Design review of the part built by this model. Coordinates are the model's own, in mm. A direction names the side the tool comes from. Coordinates: 2 decimals unless noted, no trailing zeros. Order: outer loops, then holes, each group sorted by start corner. A loop starts at its lowest first (then second) coordinate and runs counter-clockwise, first axis right, second up. Notation, with made-up numbers: (-14.75, -19) - (38.25, -19) arc R24 cw to (38.25, 11) - close; hole circle Ø9 at (68, 15.5). An arc over 180 degrees is marked (long way). Write each question's results on one line, items separated by ' | '. Start each with the question number.
```python
from build123d import *

# Parameters (mm, degrees)
F1_DEPTH = 15
F2_R     = 3.5
F3_DEPTH = 4.1
F4_R     = 2.25
F5_DEPTH = 25
F6_W     = 9.15
F6_H     = 11
F7_DEPTH = 52.92131


with BuildPart() as f1:
    # F0 (on Front) → F1 (new body)
    with BuildSketch(Plane.XZ):
        with BuildLine():
            Line((32, 0), (0, 0))
            Line((0, 0), (0, -11))
            ThreePointArc((0, -11), (0.87868, -13.12132), (3, -14))
            Line((3, -14), (6.5, -14))
            ThreePointArc((6.5, -14), (8.62132, -14.87868), (9.5, -17))
            Line((9.5, -17), (9.5, -17.757359))
            ThreePointArc((9.5, -17.757359), (9.728361, -18.90541), (10.37868, -19.87868))
            Line((10.37868, -19.87868), (26.29899, -35.79899))
            ThreePointArc((26.29899, -35.79899), (26.949308, -36.77226), (27.17767, -37.92031))
            Line((27.17767, -37.92031), (27.17767, -41.92031))
            ThreePointArc((27.17767, -41.92031), (28.056349, -44.041631), (30.17767, -44.92031))
            Line((30.17767, -44.92031), (49.92031, -44.92031))
            ThreePointArc((49.92031, -44.92031), (52.041631, -44.041631), (52.92031, -41.92031))
            Line((52.92031, -41.92031), (52.92031, -40.42031))
            ThreePointArc((52.92031, -40.42031), (52.041631, -38.29899), (49.92031, -37.42031))
            Line((49.92031, -37.42031), (44.162951, -37.42031))
            ThreePointArc((44.162951, -37.42031), (43.014901, -37.191949), (42.041631, -36.541631))
            Line((42.041631, -36.541631), (25.37868, -19.87868))
            ThreePointArc((25.37868, -19.87868), (24.728361, -18.90541), (24.5, -17.757359))
            Line((24.5, -17.757359), (24.5, -17))
            ThreePointArc((24.5, -17), (25.37868, -14.87868), (27.5, -14))
            Line((27.5, -14), (29, -14))
            ThreePointArc((29, -14), (31.12132, -13.12132), (32, -11))
            Line((32, -11), (32, 0))
        make_face()
    extrude(amount=F1_DEPTH)

    # F2 (on face) → F3 (cut)
    with BuildSketch(Plane.XZ.offset(15)):
        with Locations((26.5, -6.5)):
            Circle(F2_R)
        with Locations((5.5, -6.5)):
            Circle(F2_R)
    extrude(amount=-F3_DEPTH, mode=Mode.SUBTRACT)

    # F4 (on face) → F5 (cut)
    with BuildSketch(Plane.XZ.offset(15)):
        with Locations((5.5, -6.5)):
            Circle(F4_R)
        with Locations((26.5, -6.5)):
            Circle(F4_R)
    extrude(amount=-F5_DEPTH, mode=Mode.SUBTRACT)

    # F6 (on face) → F7 (cut, through all)
    with BuildSketch(Plane(origin=(0, 0, 0), x_dir=(0, -1, 0), z_dir=(-1, 0, 0))):
        with Locations((4.575, -5.5)):
            Rectangle(F6_W, F6_H)
        with BuildLine():
            ThreePointArc((6, -45), (6.87868, -47.12132), (9, -48))
            Line((9, -48), (15, -48))
            Line((15, -48), (15, -16))
            Line((15, -16), (9, -16))
            ThreePointArc((9, -16), (6.87868, -16.87868), (6, -19))
            Line((6, -19), (6, -45))
        make_face()
    extrude(amount=-F7_DEPTH, mode=Mode.SUBTRACT)


solid = f1.part
```
(1) Take a section at B-B (z = -6.5). State the section outline as (x, y) points.
(2) Clearance check with flat-ended pins moving along their axes: pin 1 (3.5 mm diameter, centred on x = 25.5, z = -6, fed in from -Y); pin 2 (2 mm diameter, centred on y = -6.5, z = -12, fed in from -X); pin 3 (1.7 mm diameter, centred on x = 46.5, y = -2.5, fed in from +Z); pin 4 (1.8 mm diameter, centred on x = 5, y = -4.5, fed in from -Z). State where each tip first meets the part, or that it passes through.
(3) Take a section at A-A (x = 5.5). State the section outline as (y, z) points, plus the area to 3 significant figures.
(4) Take a section at D-D (z = -34). State the section outline as (x, y) points.
(5) Mouldability with a two-part tool opening along X and no side actions: class faces 1 (the face through (7.646, -10.037, -5.824)), 2 (the face through (26.943, -2.958, -36.757)), 3 (the face through (24.735, -3.091, -18.921)) as +X half, -X half, draft (parallel to the pull), parting line (faces both ways), or undercut.
(6) To check wall thickness, follow line 1 along Z through (x, y) = (5.5, -10.1); line 2 along Y through (x, z) = (12, -10.5); line 3 along Y through (x, z) = (18.5, -21.5). State the ranges of each line that lie inside material, in increasing order. Write a range as [from, to].
(7) Tool access review of faces 4 (the face through (16, -5, -11)), 5 (the face through (5, -10.9, -9)), 6 (the face through (17, -12, -16)), 7 (the face through (28, -7, -14)): name each direction out of +Z, -Z, +X, -X, +Y, -Y from which nothing blocks a thin tool from reaching the whole face with its end or side.
(8) Take a section at C-C (y = -4.5). State the section outline as (x, z) points.
Worked out:
1) outline: (0, -15) - (2, -15) - (2, -10.9) - (3.25, -10.9) - (3.25, -9.15) - (0, -9.15) - close; (7.75, -10.9) - (9, -10.9) - (9, -15) - (23, -15) - (23, -10.9) - (24.25, -10.9) - (24.25, -9.15) - (7.75, -9.15) - close; (28.75, -10.9) - (30, -10.9) - (30, -15) - (32, -15) - (32, -9.15) - (28.75, -9.15) - close
2) pin 1: y = -10.9 | pin 2: x = 0 | pin 3: z = -37.42 | pin 4: z = -14
3) outline: (-15, -14) - (0, -14) - (0, -11) - (-9.15, -11) - (-9.15, -8.75) - (-10.9, -8.75) - (-10.9, -10) - (-15, -10) - close; (-15, -3) - (-10.9, -3) - (-10.9, -4.25) - (-9.15, -4.25) - (-9.15, 0) - (-15, 0) - close | area: 72.8 mm^2
4) outline: (24.5, -6) - (39.5, -6) - (39.5, 0) - (24.5, 0) - close
5) face 1: undercut | face 2: -X half | face 3: +X half
6) line 1: [-14, -8.75], [-4.25, 0] | line 2: [-15, -9.15] | line 3: [-6, 0]
7) face 4: +Z, +X, -X, +Y | face 5: -Y | face 6: -Z, +X, -X, -Y | face 7: +X, +Y, -Y
8) outline: (0, -11) arc R3 ccw to (3, -14) - (6.5, -14) arc R3 cw to (9.5, -17) - (9.5, -17.76) arc R3 ccw to (10.38, -19.88) - (26.3, -35.8) arc R3 cw to (27.18, -37.92) - (27.18, -41.92) arc R3 ccw to (30.18, -44.92) - (49.92, -44.92) arc R3 ccw to (52.92, -41.92) - (52.92, -40.42) arc R3 ccw to (49.92, -37.42) - (44.16, -37.42) arc R3 cw to (42.04, -36.54) - (25.38, -19.88) arc R3 cw to (24.5, -17.76) - (24.5, -17) arc R3 cw to (27.5, -14) - (29, -14) arc R3 ccw to (32, -11) - close
